Work out the finished part from the listing and answer in its coordinate system (mm). A direction names the side the tool comes from. Round coordinates to 2 decimals unless told otherwise and drop trailing zeros. Write each loop counter-clockwise with the first axis right and the second up, starting at its lowest first coordinate (ties: lowest second). Pieces come first, ordered by that corner, then holes. Notation, with made-up numbers: (25, -10.75) - (78, -10.75) arc R22 ccw to (78, 14.25) - close; hole circle Ø4 at (-1, -26.5). An arc over 180 degrees is marked (long way). Write item = value, one per line. Start each with the question number.
from build123d import *

# Parameters (mm, degrees)
SKETCH1_W           = 25.4
SKETCH1_H           = 25.4
SKETCH1_W_2         = 20.32
SKETCH1_H_2         = 20.32
EXTRUDE_THIN1_DEPTH = 254
SKETCH2_R           = 3.175
CUT_EXTRUDE1_DEPTH  = 26.4
SKETCH3_R           = 6.35
CUT_EXTRUDE2_DEPTH  = 26.4
SKETCH4_R           = 2.4892
CUT_EXTRUDE3_DEPTH  = 26.4


with BuildPart() as part:
    # Sketch1 → Extrude-Thin1 (new body, symmetric)
    with BuildSketch(Plane.XY):
        Rectangle(SKETCH1_W, SKETCH1_H)
        Rectangle(SKETCH1_W_2, SKETCH1_H_2, mode=Mode.SUBTRACT)
    extrude(amount=EXTRUDE_THIN1_DEPTH, both=True)

    # Sketch2 → Cut-Extrude1 (cut, through all)
    with BuildSketch(Plane(origin=(0, 12.7, 0), x_dir=(1, 0, 0), z_dir=(0, 1, 0))):
        with Locations((0, 241.3)):
            Circle(SKETCH2_R)
        with Locations((0, 190.5)):
            Circle(SKETCH2_R)
    extrude(amount=-CUT_EXTRUDE1_DEPTH, mode=Mode.SUBTRACT)

    # Sketch3 → Cut-Extrude2 (cut, through all)
    with BuildSketch(Plane(origin=(0, 12.7, 0), x_dir=(1, 0, 0), z_dir=(0, 1, 0))):
        with Locations((0, -228.6)):
            Circle(SKETCH3_R)
    extrude(amount=-CUT_EXTRUDE2_DEPTH, mode=Mode.SUBTRACT)

    # Sketch4 → Cut-Extrude3 (cut, through all)
    with BuildSketch(Plane.ZY.offset(12.7)):
        with Locations((-241.3, 0)):
            Circle(SKETCH4_R)
        with Locations((-203.2, 0)):
            Circle(SKETCH4_R)
    extrude(amount=-CUT_EXTRUDE3_DEPTH, mode=Mode.SUBTRACT)


solid = part.part
1. Which of the six approach directions +Z, -Z, +X, -X, +Y, -Y give full straight-line access (tool end or side, diameter ignored) to faces 5 (the face through (-10.16, 0, 4)), 6 (the face through (11, 0, -254))?
2. For a pull along Y with two mould halves and no side action, classify faces 1 (the face through (-1.38, -11.41, 234.8)), 2 (the face through (0, -10.16, 4)), 3 (the face through (0, 12.7, 4)), 4 (the face through (10.16, 0, 4)) as released by +Y, released by -Y, zero draft, split by the parting line, or undercut.
3. Consider line 1 (Z direction, x = 0, y = -11.45) (3 decimals); line 2 (X direction, y = -6.25, z = 202). Determine where each line is inside the solid, lowest interval first.
4. Find section B-B on z = -20.5. Give the vertices of the cut face in (x, y), plus the area to 3 significant figures.
5. Find section A-A on z = 228.6. Give the vertices of the cut face in (x, y), plus the area to 3 significant figures.
6. This flat-tipped pin is pushed along its axis until it touches: pin 1 (8 mm diameter, centred on y = 0, z = -241.3, fed in from +X). Where does it stop, or does it pass through?
Answer key:
q1.face_5 = +Z, -Z
q1.face_6 = -Z, +X, -X, +Y, -Y
q2.face_1 = zero draft
q2.face_2 = undercut
q2.face_3 = released by +Y
q2.face_4 = undercut
q3.line_1 = -254 to -244.475, -238.125 to -193.675, -187.325 to 222.25, 234.95 to 254
q3.line_2 = -12.7 to -10.16, 10.16 to 12.7
q4.outline = (-12.7, -12.7) - (12.7, -12.7) - (12.7, 12.7) - (-12.7, 12.7) - close; hole (-10.16, -10.16) - (10.16, -10.16) - (10.16, 10.16) - (-10.16, 10.16) - close
q4.area = 232 mm²
q5.outline = (-12.7, -12.7) - (-6.35, -12.7) - (-6.35, -10.16) - (-10.16, -10.16) - (-10.16, 10.16) - (-6.35, 10.16) - (-6.35, 12.7) - (-12.7, 12.7) - close; (6.35, -12.7) - (12.7, -12.7) - (12.7, 12.7) - (6.35, 12.7) - (6.35, 10.16) - (10.16, 10.16) - (10.16, -10.16) - (6.35, -10.16) - close
q5.area = 168 mm²
q6.pin_1 = 12.7
